from build123d import *

# Parameters (mm, degrees)
F1_DEPTH = 635
F3_D     = 177.8


with BuildPart() as f1:
    # F0 (on Front) → F1 (new body)
    with BuildSketch(Plane.XZ):
        Polygon((0, 254), (0, 0), (762, 0), (762, 254), (508, 254), (508, 317.5), (254, 317.5), (254, 254), align=None)
    extrude(amount=-F1_DEPTH)

    # F3 (through all)
    with Locations(Plane.XY.offset(317.5)):
        with Locations((381, 317.5)):
            Hole(F3_D / 2)


solid = f1.part
The model under review builds one solid part; all positions refer to its coordinate system, in mm. A direction names the side the tool comes from. Coordinates: 2 decimals unless noted, no trailing zeros. Write each loop counter-clockwise with the first axis right and the second up, starting at its lowest first coordinate (ties: lowest second). Pieces come first, ordered by that corner, then holes. Notation, with made-up numbers: (81.5, -27.75) - (109.5, -27.75) arc R20 ccw to (109.5, 3.25) - close; hole circle Ø9 at (12, 27). An arc over 180 degrees is marked (long way). Answer as CSV lines item,"result".
(1) Tool access review of faces 4 (the flat face through (0, 313, 129)), 5 (the flat face through (637, 313, 254)), 6 (the flat face through (129, 313, 254)): name each direction out of +Z, -Z, +X, -X, +Y, -Y from which nothing blocks a thin tool from reaching the whole face with its end or side.
Data:
face 4,"+Z, -Z, -X, +Y, -Y"
face 5,"+Z, +X, +Y, -Y"
face 6,"+Z, -X, +Y, -Y"
(2) We need section C-C (x = 381). Give the boundary of the cut face in (y, z).
Data:
outline,"(0, 0) - (228.6, 0) - (228.6, 317.5) - (0, 317.5) - close; (406.4, 0) - (635, 0) - (635, 317.5) - (406.4, 317.5) - close"
(3) For line 1 along Y through (x, z) = (381, 84); line 2 along X through (y, z) = (317, 164); line 3 along Z through (x, y) = (173.5, 128), list the stretches that pass through material, from the lowest coordinate up. Write a range as [from, to].
Data:
line 1,"y = [0, 228.6], [406.4, 635]"
line 2,"x = [0, 292.1], [469.9, 762]"
line 3,"z = [0, 254]"
(4) We need section A-A (y = 317.5). Give the boundary of the cut face in (x, z).
Data:
outline,"(0, 0) - (292.1, 0) - (292.1, 317.5) - (254, 317.5) - (254, 254) - (0, 254) - close; (469.9, 0) - (762, 0) - (762, 254) - (508, 254) - (508, 317.5) - (469.9, 317.5) - close"
(5) We need section D-D (y = 455.5). Give the boundary of the cut face in (x, z).
Data:
outline,"(0, 0) - (762, 0) - (762, 254) - (508, 254) - (508, 317.5) - (254, 317.5) - (254, 254) - (0, 254) - close"
(6) Clearance check with a flat-ended pin moving along its axis: pin 1 Ø3 at (y, z) = (146, 102.5) entering from -X. State where the tip first meets the part, or that it passes through.
Data:
pin 1,"stops at x = 0"
(7) Mouldability with a two-part tool opening along X and no side actions: class faces 1 (the flat face through (376, 0, 126)), 2 (the flat face through (254, 313, 286)), 3 (the cylindrical face through (298.88, 283.45, 156.53)) as pulls with the +X half, pulls with the -X half, needs draft (parallel to the pull), parting line crosses it, or undercut.
Data:
face 1,"needs draft"
face 2,"pulls with the -X half"
face 3,"undercut"
(8) We need section B-B (z = 275.5). Give the boundary of the cut face in (x, y), plus the area to 3 significant figures.
Data:
outline,"(254, 0) - (508, 0) - (508, 635) - (254, 635) - close; hole circle Ø177.8 at (381, 317.5)"
area,"136,000 mm2"
